Here's the drawing with two shaded views (mm, measured from the low corner). I have some questions. A direction names the side the tool comes from. Round coordinates to 2 decimals unless told otherwise and drop trailing zeros. Loops run counter-clockwise (first coordinate to the right, second up) from the corner with the lowest first, then second, coordinate; pieces in that order, holes last.
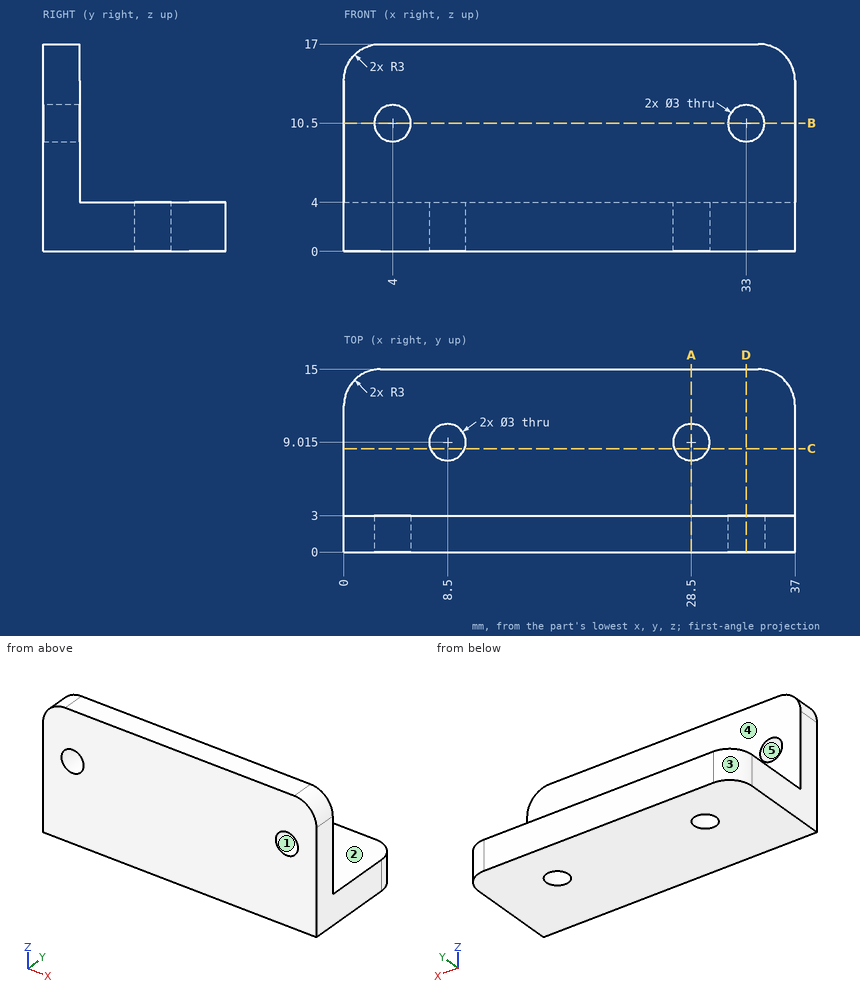
Item 1: For the marked faces 4 and 5, which set-ups out of +Z, -Z, +X, -X, +Y, -Y let a thin tool reach every point of the face, with its end or its side?
Results list:
face 4: +Z, +X, -X, +Y
face 5: +Y, -Y
Item 2: If we section it at C-C, the plane y = 8.5: Please give me the cut outline in (x, z).
Results list:
outline: (0, 0) - (7.09, 0) - (7.09, 4) - (0, 4) - close; (9.91, 0) - (27.09, 0) - (27.09, 4) - (9.91, 4) - close; (29.91, 0) - (37, 0) - (37, 4) - (29.91, 4) - close
Item 3: If I drill on line 1 along X through (y, z) = (1.85, 10.5); line 2 along Z through (x, y) = (18, 12.5); line 3 along Y through (x, z) = (32.5, 5), over which ranges is the centre line in solid material (lowest first)?
Results list:
line 1: x = 0 to 2.5, 5.5 to 31.5, 34.5 to 37
line 2: z = 0 to 4
line 3: y = 0 to 3
Item 4: If we section it at B-B, the plane z = 10.5: Please give me the cut outline in (x, y).
Results list:
outline: (0, 0) - (2.5, 0) - (2.5, 3) - (0, 3) - close; (5.5, 0) - (31.5, 0) - (31.5, 3) - (5.5, 3) - close; (34.5, 0) - (37, 0) - (37, 3) - (34.5, 3) - close
Item 5: Will these pins go through, and if not, where does the flat tip stop? pin 1 (2 mm diameter, centred on x = 6, z = 14, fed in from +Y); pin 2 (3.5 mm diameter, centred on x = 19, y = 11, fed in from +Z).
Results list:
pin 1: stops at y = 3
pin 2: stops at z = 4
Item 6: We'd pull the mould along Z, two halves only. Please class the marked faces 1, 2 and 3: released by +Z, released by -Z, zero draft, split by the parting line, or undercut.
Results list:
face 1: undercut
face 2: released by +Z
face 3: zero draft
Item 7: If we section it at A-A, the plane x = 28.5: Please give me the cut outline in (y, z) (1 decimal), then the cut area to 3 significant figures.
Results list:
outline: (0, 0) - (7.5, 0) - (7.5, 4) - (3, 4) - (3, 17) - (0, 17) - close; (10.5, 0) - (15, 0) - (15, 4) - (10.5, 4) - close
area: 87.0 mm2
Item 8: If we section it at D-D, the plane x = 33: Please give me the cut outline in (y, z).
Results list:
outline: (0, 0) - (15, 0) - (15, 4) - (3, 4) - (3, 9) - (0, 9) - close; (0, 12) - (3, 12) - (3, 17) - (0, 17) - close
